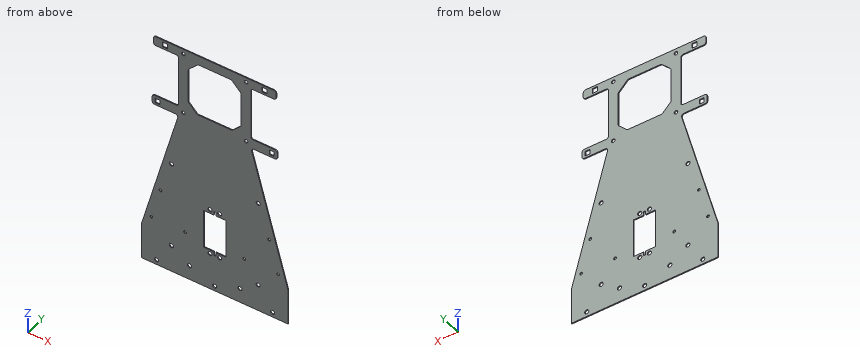
```python
from build123d import *

# Parameters (mm, degrees)
SKETCH26_R          = 1.875
SKETCH26_W          = 5
SKETCH26_H          = 5
SKETCH26_R_2        = 2.15
SKETCH26_R_3        = 1.45
BOSS_EXTRUDE6_DEPTH = 1


with BuildPart() as part:
    # Sketch26 → Boss-Extrude6 (new body)
    with BuildSketch(Plane(origin=(0, 0, 0), x_dir=(1, 0, 0), z_dir=(0, 1, 0))):
        with BuildLine():
            Line((76.013272408, 51.623832483), (76.013272408, 88.823544949))
            Line((76.013272408, 88.823544949), (-76.102081629, 88.823544949))
            Line((-76.102081629, 88.823544949), (-76.102081629, 51.776273242))
            Line((-76.102081629, 51.776273242), (-38.382791234, -83.527277546))
            ThreePointArc((-38.382791234, -83.527277546), (-38.800395788, -85.710062519), (-40.791178841, -86.69785128))
            Line((-40.791178841, -86.69785128), (-62.37853755, -86.69785128))
            ThreePointArc((-62.37853755, -86.69785128), (-64.146304503, -87.430084327), (-64.87853755, -89.19785128))
            Line((-64.87853755, -89.19785128), (-64.87853755, -94.216442532))
            ThreePointArc((-64.87853755, -94.216442532), (-64.146304503, -95.984209485), (-62.37853755, -96.716442532))
            Line((-62.37853755, -96.716442532), (-40, -96.716442532))
            ThreePointArc((-40, -96.716442532), (-38.232233047, -97.448675579), (-37.5, -99.216442532))
            Line((-37.5, -99.216442532), (-37.5, -149.615103737))
            ThreePointArc((-37.5, -149.615103737), (-38.232233047, -151.38287069), (-40, -152.115103737))
            Line((-40, -152.115103737), (-61.156929158, -152.115103737))
            ThreePointArc((-61.156929158, -152.115103737), (-62.924696111, -152.847336784), (-63.656929158, -154.615103737))
            Line((-63.656929158, -154.615103737), (-63.656929158, -159.216442532))
            ThreePointArc((-63.656929158, -159.216442532), (-62.924696111, -160.984209485), (-61.156929158, -161.716442532))
            Line((-61.156929158, -161.716442532), (-34.988305588, -161.716442532))
            Line((-34.988305588, -161.716442532), (-29.988305588, -161.716442532))
            Line((-29.988305588, -161.716442532), (30, -161.716442532))
            Line((30, -161.716442532), (61.156929158, -161.716442532))
            ThreePointArc((61.156929158, -161.716442532), (62.924696111, -160.984209485), (63.656929158, -159.216442532))
            Line((63.656929158, -159.216442532), (63.656929158, -154.615103737))
            ThreePointArc((63.656929158, -154.615103737), (62.924696111, -152.847336784), (61.156929158, -152.115103737))
            Line((61.156929158, -152.115103737), (40, -152.115103737))
            ThreePointArc((40, -152.115103737), (38.232233047, -151.38287069), (37.5, -149.615103737))
            Line((37.5, -149.615103737), (37.5, -99.216442532))
            ThreePointArc((37.5, -99.216442532), (38.232233047, -97.448675579), (40, -96.716442532))
            Line((40, -96.716442532), (62.37853755, -96.716442532))
            ThreePointArc((62.37853755, -96.716442532), (64.146304503, -95.984209485), (64.87853755, -94.216442532))
            Line((64.87853755, -94.216442532), (64.87853755, -89.19785128))
            ThreePointArc((64.87853755, -89.19785128), (64.146304503, -87.430084327), (62.37853755, -86.69785128))
            Line((62.37853755, -86.69785128), (40.791178841, -86.69785128))
            ThreePointArc((40.791178841, -86.69785128), (38.800395788, -85.710062519), (38.382791234, -83.527277546))
            Line((38.382791234, -83.527277546), (75.505468817, 49.800039197))
            Line((75.505468817, 49.800039197), (76.013272408, 51.623832483))
        make_face()
        Polygon((-54.2, -154.243772746), (-49, -154.243772746), (-49, -159.443772746), (-54.2, -159.443772746), (-54.2, -156.286487859), align=None, mode=Mode.SUBTRACT)
        with Locations((-32.5, -156.716442532)):
            Circle(SKETCH26_R, mode=Mode.SUBTRACT)
        with Locations((-59.2, -91.39597875)):
            Rectangle(SKETCH26_W, SKETCH26_H, mode=Mode.SUBTRACT)
        with Locations((-32.5, -91.716442532)):
            Circle(SKETCH26_R, mode=Mode.SUBTRACT)
        with Locations((32.5, -156.716442532)):
            Circle(SKETCH26_R, mode=Mode.SUBTRACT)
        with BuildLine():
            Line((27.5, -107.101933172), (27.5, -140.94514821))
            ThreePointArc((27.5, -140.94514821), (27.309376305, -141.902635067), (26.766575135, -142.714106178))
            Line((26.766575135, -142.714106178), (18.084925196, -151.384061705))
            ThreePointArc((18.084925196, -151.384061705), (17.274280257, -151.925124832), (16.318350061, -152.115103737))
            Line((16.318350061, -152.115103737), (-16.318350061, -152.115103737))
            ThreePointArc((-16.318350061, -152.115103737), (-17.275058642, -151.924802568), (-18.086117014, -151.38287069))
            Line((-18.086117014, -151.38287069), (-26.764204101, -142.704783602))
            ThreePointArc((-26.764204101, -142.704783602), (-27.306229203, -141.89350014), (-27.496437101, -140.936529386))
            Line((-27.496437101, -140.936529386), (-27.489840484, -107.09128644))
            ThreePointArc((-27.489840484, -107.09128644), (-27.299446118, -106.134840041), (-26.757607485, -105.324006751))
            Line((-26.757607485, -105.324006751), (-18.882276313, -97.448675579))
            ThreePointArc((-18.882276313, -97.448675579), (-18.071217941, -96.906743701), (-17.11450936, -96.716442532))
            Line((-17.11450936, -96.716442532), (17.11450936, -96.716442532))
            ThreePointArc((17.11450936, -96.716442532), (18.071217941, -96.906743701), (18.882276313, -97.448675579))
            Line((18.882276313, -97.448675579), (26.767766953, -105.334166219))
            ThreePointArc((26.767766953, -105.334166219), (27.309698831, -106.145224591), (27.5, -107.101933172))
        make_face(mode=Mode.SUBTRACT)
        Polygon((54.2, -159.443772746), (49, -159.443772746), (49, -154.243772746), (54.2, -154.243772746), (54.2, -156.286487859), align=None, mode=Mode.SUBTRACT)
        with Locations((32.5, -91.716442532)):
            Circle(SKETCH26_R, mode=Mode.SUBTRACT)
        with Locations((59.2, -91.39597875)):
            Rectangle(SKETCH26_W, SKETCH26_H, mode=Mode.SUBTRACT)
        with Locations((-44.91002895, -29.282587791)):
            Circle(SKETCH26_R_2, mode=Mode.SUBTRACT)
        with Locations((-56.275133419, 5.22710987)):
            Circle(SKETCH26_R_3, mode=Mode.SUBTRACT)
        with Locations((-4.91002895, 1.717412209)):
            Circle(SKETCH26_R_2, mode=Mode.SUBTRACT)
        with Locations((-65.710275059, 38.931384113)):
            Circle(SKETCH26_R_3, mode=Mode.SUBTRACT)
        with Locations((-60.263272408, 83.747616616)):
            Circle(SKETCH26_R_2, mode=Mode.SUBTRACT)
        with Locations((-44.91002895, 60.717412209)):
            Circle(SKETCH26_R_2, mode=Mode.SUBTRACT)
        with Locations((-30.728022224, 38.916998548)):
            Circle(SKETCH26_R_3, mode=Mode.SUBTRACT)
        with Locations((-4.91002895, 50.217412209)):
            Circle(SKETCH26_R_2, mode=Mode.SUBTRACT)
        with Locations((-26.102081629, 73.823544949)):
            Circle(SKETCH26_R_2, mode=Mode.SUBTRACT)
        with Locations((5.08997105, 1.717412209)):
            Circle(SKETCH26_R_2, mode=Mode.SUBTRACT)
        Polygon((11.577692982, 46.217412209), (11.577692982, 5.717412209), (1.08997105, 5.717412209), (1.08997105, 1.717412209), (-0.91002895, 1.717412209), (-0.91002895, 5.717412209), (-11.397750883, 5.717412209), (-11.397750883, 46.217412209), (-0.91002895, 46.217412209), (-0.91002895, 50.217412209), (1.08997105, 50.217412209), (1.08997105, 46.217412209), align=None, mode=Mode.SUBTRACT)
        with Locations((45.08997105, -29.282587791)):
            Circle(SKETCH26_R_2, mode=Mode.SUBTRACT)
        with Locations((56.339989947, 5.199572045)):
            Circle(SKETCH26_R_3, mode=Mode.SUBTRACT)
        with Locations((5.08997105, 50.217412209)):
            Circle(SKETCH26_R_2, mode=Mode.SUBTRACT)
        with Locations((30.728022224, 38.916998548)):
            Circle(SKETCH26_R_3, mode=Mode.SUBTRACT)
        with Locations((0, 83.74802142)):
            Circle(SKETCH26_R_2, mode=Mode.SUBTRACT)
        with Locations((26.102081629, 73.823544949)):
            Circle(SKETCH26_R_2, mode=Mode.SUBTRACT)
        with Locations((65.728022224, 38.916998548)):
            Circle(SKETCH26_R_3, mode=Mode.SUBTRACT)
        with Locations((45.08997105, 60.717412209)):
            Circle(SKETCH26_R_2, mode=Mode.SUBTRACT)
        with Locations((59.999999999, 83.747618385)):
            Circle(SKETCH26_R_2, mode=Mode.SUBTRACT)
    extrude(amount=BOSS_EXTRUDE6_DEPTH)


solid = part.part
```
Verification items for the finished model (mm, model axes). Give positions to 0.01 mm unless a question says otherwise; leave off trailing zeros. Loops run counter-clockwise (first coordinate to the right, second up) from the corner with the lowest first, then second, coordinate; pieces in that order, holes last.
1. Section check B-B, the plane y = 0.4. Count the separate pieces of the cut face and the enclosed holes in it, then the cut area to 3 significant figures.
2. Go/stop test with flat-tipped pins: pin 1 Ø0.5 at (y, z) = (0.5, 157) entering from +X; pin 2 Ø0.5 at (y, z) = (0.5, 123) entering from -X; pin 3 Ø0.5 at (y, z) = (0.5, -17.5) entering from +X. Record where each tip stops, or that it passes through.
3. Thickness scan on line 1 (Z direction, x = 10, y = 0.4); line 2 (Z direction, x = -32.5, y = 0.45); line 3 (Z direction, x = 15, y = 0.85). Record the ranges inside material, lowest first.
4. Section check D-D, the plane z = 13. Enter the section's corners in (x, y).
5. Section check A-A, the plane z = 117.5. Enter the section's corners in (x, y).
6. Section check C-C, the plane z = -26.5. Enter the section's corners in (x, y), then the cut area to 3 significant figures.
Geometry says:
1. separate pieces: 1
1. enclosed holes: 29
1. area: 23,900 mm2
2. pin 1: stops at x = 63.66
2. pin 2: stops at x = -37.5
2. pin 3: stops at x = 66.58
3. line 1: z = -88.82 to -46.22, -5.72 to 96.72, 152.12 to 161.72
3. line 2: z = -88.82 to 89.84, 93.59 to 154.84, 158.59 to 161.72
3. line 3: z = -88.82 to 96.72, 152.12 to 161.72
4. outline: (-58.04, 0) - (58.02, 0) - (58.02, 1) - (-58.04, 1) - close
5. outline: (-37.5, 0) - (-27.49, 0) - (-27.49, 1) - (-37.5, 1) - close; (27.5, 0) - (37.5, 0) - (37.5, 1) - (27.5, 1) - close
6. outline: (-69.06, 0) - (-11.4, 0) - (-11.4, 1) - (-69.06, 1) - close; (11.58, 0) - (69.02, 0) - (69.02, 1) - (11.58, 1) - close
6. area: 115 mm2
